Part print with two shaded views. Sizes in mm from the minimum x, y, z corner. A direction names the side the tool comes from. Round coordinates to 2 decimals unless told otherwise and drop trailing zeros. Loops run counter-clockwise (first coordinate to the right, second up) from the corner with the lowest first, then second, coordinate; pieces in that order, holes last. Notation, with made-up numbers: (1, 74.5) -> (52, 74.5) arc R21 cw to (52, 79.5) -> close; hole circle Ø4 at (-28.75, 75.25). An arc over 180 degrees is marked (long way). Use a Markdown table: item, result. Add a question column.
Item 1: Probe line 1 (Z direction, x = 3.1, y = 0.7); line 2 (Y direction, x = 3, z = 1.05); line 3 (Y direction, x = 3, z = 0.6). List the from-to ranges inside material, lowest first. Write a range as [from, to].
Item 2: Cut at A-A, the plane y = 3. List the corners of the cut face in (x, z), plus the area to 3 significant figures.
Item 3: Which spindle directions (+Z, -Z, +X, -X, +Y, -Y) get a long thin tool onto all of the face, cutting with end or side? Do the marked faces 4 and 5. Say none if no direction does.
Item 4: Cut at D-D, the plane y = 4.8. List the corners of the cut face in (x, z), plus the area to 3 significant figures.
Item 5: Cut at C-C, the plane z = 0.2. List the corners of the cut face in (x, y).
Item 6: Two-plate mould, pull along X, no slides. Class the marked faces 1, 2 and 3: pulls with the +X half, pulls with the -X half, needs draft (parallel to the pull), parting line crosses it, or undercut.
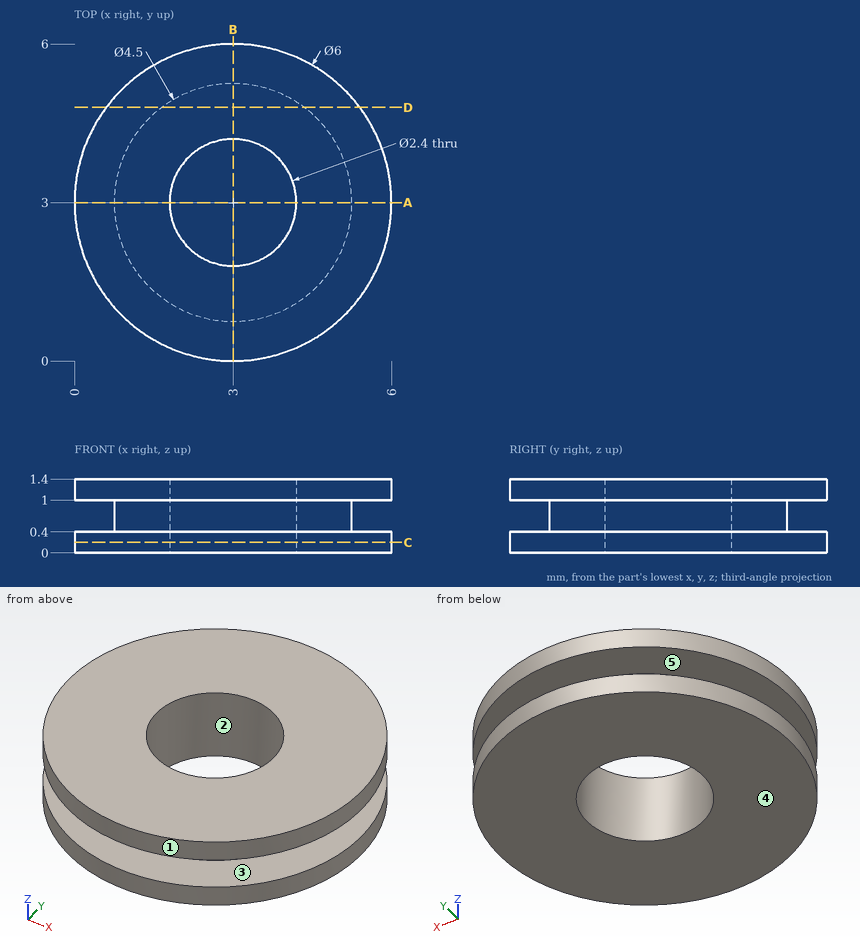
A:
| question | item | result |
|---|---|---|
| 1 | line 1 | z = [0, 0.4], [1, 1.4] |
| 1 | line 2 | y = [0, 1.8], [4.2, 6] |
| 1 | line 3 | y = [0.75, 1.8], [4.2, 5.25] |
| 2 | outline | (0, 0) -> (1.8, 0) -> (1.8, 1.4) -> (0, 1.4) -> (0, 1) -> (0.75, 1) -> (0.75, 0.4) -> (0, 0.4) -> close; (4.2, 0) -> (6, 0) -> (6, 0.4) -> (5.25, 0.4) -> (5.25, 1) -> (6, 1) -> (6, 1.4) -> (4.2, 1.4) -> close |
| 2 | area | 4.14 mm^2 |
| 3 | face 4 | -Z, +X, -X, +Y, -Y |
| 3 | face 5 | none |
| 4 | outline | (0.6, 0) -> (5.4, 0) -> (5.4, 0.4) -> (4.35, 0.4) -> (4.35, 1) -> (5.4, 1) -> (5.4, 1.4) -> (0.6, 1.4) -> (0.6, 1) -> (1.65, 1) -> (1.65, 0.4) -> (0.6, 0.4) -> close |
| 4 | area | 5.46 mm^2 |
| 5 | outline | circle Ø6 at (3, 3); hole circle Ø2.4 at (3, 3) |
| 6 | face 1 | parting line crosses it |
| 6 | face 2 | undercut |
| 6 | face 3 | needs draft |
